from build123d import *

# Parameters (mm, degrees)
CYLINDER_R        = 20.5
CYLINDER_DEPTH    = 120
CYLINDER002_R     = 26
CYLINDER002_DEPTH = 10
CHAMFER_SIZE      = 5
CYLINDER001_R     = 21
CYLINDER001_DEPTH = 100
BOX_W             = 50
BOX_H             = 50
BOX_DEPTH         = 2.5


with BuildPart() as cylinder:
    # Cylinder → Cylinder (new body)
    with BuildSketch(Plane(origin=(25, 25, 0), x_dir=(1, 0, 0), z_dir=(0, 0, 1))):
        Circle(CYLINDER_R)
    extrude(amount=CYLINDER_DEPTH)


with BuildPart() as chamfer_body:
    # Cylinder002 → Cylinder002 (new body)
    with BuildSketch(Plane(origin=(25, 25, 93.5), x_dir=(1, 0, 0), z_dir=(0, 0, 1))):
        Circle(CYLINDER002_R)
    extrude(amount=CYLINDER002_DEPTH)

    # Chamfer
    chamfer_edges = [chamfer_body.edges().sort_by_distance(p)[0] for p in [
        (-1, 25, 93.5),
    ]]
    chamfer(chamfer_edges, length=CHAMFER_SIZE)


with BuildPart() as fusion:
    # Cylinder001 → Cylinder001 (new body)
    with BuildSketch(Plane(origin=(25, 25, 0), x_dir=(1, 0, 0), z_dir=(0, 0, 1))):
        Circle(CYLINDER001_R)
    extrude(amount=CYLINDER001_DEPTH)

    # Fusion: union Chamfer body
    add(chamfer_body.part)


with BuildPart() as cut:
    # Box → Box (new body)
    with BuildSketch(Plane.XY):
        with Locations((25, 25)):
            Rectangle(BOX_W, BOX_H)
    extrude(amount=BOX_DEPTH)

    # Fusion001: union Fusion
    add(fusion.part)

    # Cut: cut Cylinder
    add(cylinder.part, mode=Mode.SUBTRACT)


solid = cut.part
Geometry check sheet. Reference: the model listing, model coordinates, mm. A direction names the side the tool comes from. Coordinates: 2 decimals unless noted, no trailing zeros. Order: outer loops, then holes, each group sorted by start corner. A loop starts at its lowest first (then second) coordinate and runs counter-clockwise, first axis right, second up. Notation, with made-up numbers: M -37,47.5 L -10,47.5 A25 ccw -10,84.5 Z; hole C 42,10.25 d8. An arc over 180 degrees is marked long. Use CSV: the item, a comma, the result in double quotes.
Item 1: Mould release check, pull along X, two halves, no side actions. Record for faces 4 (the flat face through (47, 25, 2.5)), 5 (the conical face through (44.62, 16.86, 93.74)), 6 (the cylindrical face through (4.52, 25.9, 51.03)): pulls with the +X half, pulls with the -X half, needs draft (parallel to the pull), parting line crosses it, or undercut.
Returned:
face 4,"needs draft"
face 5,"parting line crosses it"
face 6,"undercut"
Item 2: Thickness scan on line 1 along X through (y, z) = (25, 50.5); line 2 along X through (y, z) = (9, 4). Record the ranges inside material, lowest first.
Returned:
line 1,"x = 4 to 4.5, 45.5 to 46"
line 2,"x = 11.4 to 12.18, 37.82 to 38.6"
Item 3: Cross-section at C-C on z = 50. Record the cut outline in (x, y).
Returned:
outline,"C 25,25 d42; hole C 25,25 d41"
Item 4: Cross-section at A-A on x = 25. Record the cut outline in (y, z).
Returned:
outline,"M -1,98.5 L 4,93.5 L 4,2.5 L 0,2.5 L 0,0 L 4.5,0 L 4.5,103.5 L -1,103.5 Z; M 45.5,0 L 50,0 L 50,2.5 L 46,2.5 L 46,93.5 L 51,98.5 L 51,103.5 L 45.5,103.5 Z"
Item 5: Tool access check on faces 1 (the flat face through (0, 25, 1)), 2 (the cylindrical face through (36.3, 42.7, 47.4)), 3 (the flat face through (50, 25, 1)). Record the directions out of +Z, -Z, +X, -X, +Y, -Y that give a thin tool (end or side, any length) a straight path to the whole face; none if there is none.
Returned:
face 1,"-Z, -X, +Y, -Y"
face 2,"none"
face 3,"-Z, +X, +Y, -Y"
Item 6: Gauge pin test, flat ends, axial feed: pin 1 Ø1.5 at (x, z) = (23.5, 81.5) entering from +Y; pin 2 Ø10 at (y, z) = (28.5, 11.5) entering from +X; pin 3 Ø0.8 at (x, z) = (14.5, 2) entering from +Y; pin 4 Ø12 at (x, y) = (15, 28.5) entering from -Z. Record the tip position at first contact, or that the pin passes through.
Returned:
pin 1,"stops at y = 45.99"
pin 2,"stops at x = 46"
pin 3,"stops at y = 50"
pin 4,"passes through"
